Source: CAD feature listing. Evaluate the final solid. Frame: model axes, mm. A direction names the side the tool comes from. Give positions to 0.01 mm unless a question says otherwise; leave off trailing zeros. Write each loop counter-clockwise with the first axis right and the second up, starting at its lowest first coordinate (ties: lowest second). Pieces come first, ordered by that corner, then holes. Notation, with made-up numbers: (-23, 80) - (-4, 80) arc R23 ccw to (-4, 114) - close; hole circle Ø4 at (71.5, 74). An arc over 180 degrees is marked (long way). Answer as a JSON object with one key per item and string values. Group by question number.
from build123d import *

# Parameters (mm, degrees)
SKETCH2_R          = 1.785
CUT_EXTRUDE1_DEPTH = 1.5


with BuildPart() as part:
    # Sketch1 → Revolve1 (revolve)
    with BuildSketch(Plane.XY, mode=Mode.PRIVATE) as revolve1_sk:
        with BuildLine():
            Line((50.583920217, 5), (0, 5))
            Line((0, 5), (0, 1.5))
            Line((0, 1.5), (47, 1.5))
            Line((47, 1.5), (47, 0))
            Line((47, 0), (56.5, 0))
            ThreePointArc((56.5, 0), (54.456903563, 3.582575695), (50.583920217, 5))
        make_face()
    revolve(revolve1_sk.sketch.rotate(Axis((0, 0, 0), (0, 1, 0)), 90), axis=Axis((0, 0, 0), (0, 1, 0)))

    # Sketch2 → Cut-Extrude1 (cut)
    with BuildSketch(Plane.XZ):
        with Locations(Location((0, 51.91, 0), (0, 0, 270))):
            Circle(SKETCH2_R)
        with Locations(Location((51.91, 0, 0), (0, 0, 270))):
            Circle(SKETCH2_R)
        with Locations(Location((0, -51.91, 0), (0, 0, 270))):
            Circle(SKETCH2_R)
        with Locations(Location((-51.91, 0, 0), (0, 0, 270))):
            Circle(SKETCH2_R)
    extrude(amount=-CUT_EXTRUDE1_DEPTH, mode=Mode.SUBTRACT)


solid = part.part
Q1. Reachability of faces 1 (the flat face through (-46, 0, -13)), 2 (the cylindrical face through (0.078, 0.74, -50.127)) from +Z, -Z, +X, -X, +Y, -Y: full face, straight path, thin tool, end or side. Return the list, or none.
Q2. First-contact query: pin 1 Ø3 at (x, z) = (-51.91, 0) entering from +Y; pin 2 Ø1 at (y, z) = (3, 36.5) entering from +X; pin 3 Ø1.1 at (x, z) = (-0.5, -52.5) entering from -Y; pin 4 Ø3 at (x, y) = (36.5, 2.5) entering from -Z. Flat tips, straight axial feed; report the tip coordinate or a pass-through.
Q3. Draft query along X for faces 3 (the flat face through (0, 1.5, 52)), 4 (the flat face through (-1, 5, 1)). Return one class per face: released by +X, released by -X, zero draft, split by the parting line, or undercut.
Q4. Section A-A on z = 0. Return the cut outline in (x, y) (3 decimals), then the cut area to 3 significant figures.
Q5. Ray query, probe 1 along X at (y, z) = (0.3, 0) (3 decimals); probe 2 along Y at (x, z) = (37.5, -9); probe 3 along X at (y, z) = (0.4, 33). Return the intervals inside material, ascending. Write a range as [from, to].
Q6. Section B-B on y = 3.75. Return the cut outline in (x, z), then the cut area to 3 significant figures.
Taken from the geometry:
{
 "1": {"face 1": "+Z, -Z, +X, -X, -Y", "face 2": "-Y"},
 "2": {"pin 1": "stops at y = 5", "pin 2": "stops at x = 41.92", "pin 3": "stops at y = 1.5", "pin 4": "stops at z = -43.46"},
 "3": {"face 3": "undercut", "face 4": "zero draft"},
 "4": {"outline": "(-56.5, 0) - (-53.695, 0) - (-53.695, 1.5) - (-50.125, 1.5) - (-50.125, 0) - (-47, 0) - (-47, 1.5) - (47, 1.5) - (47, 0) - (50.125, 0) - (50.125, 1.5) - (53.695, 1.5) - (53.695, 0) - (56.5, 0) arc R6 ccw to (50.584, 5) - (-50.584, 5) arc R6 ccw to start", "area": "399 mm²"},
 "5": {"probe 1": "x = [-56.441, -53.695], [-50.125, -47], [47, 50.125], [53.695, 56.441]", "probe 2": "y = [1.5, 5]", "probe 3": "x = [-45.76, -33.47], [33.47, 45.76]"},
 "6": {"outline": "circle Ø108.5 at (0, 0)", "area": "9,250 mm²"}
}
